Solid Edge part; units mm, degrees
sketch "Sketch1" plane through (-100.203, 10.668, -35.941) normal (0, 0, 1) x (-1, 0, 0)
  line L0 (4.1402, -5.9309) -> (4.1402, 5.9309)
  line L1 (4.1402, 5.9309) -> (-9.6647, 5.9309)
  line L2 (-9.6647, 5.9309) -> (-9.6647, -5.9309)
  line L3 (-9.6647, -5.9309) -> (4.1402, -5.9309)
extrude "Protrusion1" add sketch "Sketch1" along normal blind 5.334
sketch "Sketch2" plane through (-97.4407, 16.5989, -33.274) normal (0, 1, 0) x (-1, 0, 0)
  line L0 (4.9721, 2.9711) -> (3.1941, 2.9711)
  line L1 (3.1941, 2.9711) -> (3.1941, -1.3462)
  line L2 (3.1941, -1.3462) -> (4.9721, -1.3462)
  line L3 (4.9721, -1.3462) -> (4.9721, 2.9711)
extrude "Cutout1" cut sketch "Sketch2" against normal through all
sketch "Sketch3" plane through (-97.4407, 16.5989, -33.274) normal (0, 1, 0) x (-1, 0, 0)
  line L0 (0.6541, -1.6616) -> (-6.9024, -1.6616)
  line L1 (-6.9024, -1.6616) -> (-6.9024, -2.667)
  line L2 (-6.9024, -2.667) -> (0.6541, -2.667)
  line L3 (0.6541, -2.667) -> (0.6541, -1.6616)
extrude "Cutout2" cut sketch "Sketch3" against normal through all
fillet "Round_1" radius 0.8636 4 edges at (-104.3432, 10.668, -30.607) (-102.4128, 10.668, -30.607) (-100.6348, 10.668, -30.607) (-90.5383, 10.668, -30.607)
properties material "Gold"
Verification items for the finished model (mm, model axes). A direction names the side the tool comes from. Round coordinates to 2 decimals unless told otherwise and drop trailing zeros. Loops run counter-clockwise (first coordinate to the right, second up) from the corner with the lowest first, then second, coordinate; pieces in that order, holes last. Notation, with made-up numbers: (-14, 39.5) - (23, 39.5) arc R12 cw to (23, 56.5) - close; hole circle Ø8 at (-16.5, 25.25). An arc over 180 degrees is marked (long way). Answer in a Markdown table with one row per item. Add a question column.
Q1. Gauge pin test, flat ends, axial feed: pin 1 (2.5 mm diameter, centred on x = -94, y = 12, fed in from -Z); pin 2 (0.5 mm diameter, centred on x = -101, y = 10.5, fed in from +Z); pin 3 (0.8 mm diameter, centred on y = 12.5, z = -35.5, fed in from +X). Record the tip position at first contact, or that the pin passes through.
Q2. Section check B-B on y = 13. Enter the section's corners in (x, z), plus the area to 3 significant figures.
Q3. Release check for a two-part mould opening along X. For faces 1 (the face through (-97, 16.599, -33)), 2 (the face through (-102, 11, -34.62)), 3 (the face through (-104.08, 10.58, -30.85)) record: pulls with the +X half, pulls with the -X half, needs draft (parallel to the pull), parting line crosses it, or undercut.
Q4. Section check A-A on z = -34.45. Enter the section's corners in (x, y).
Q5. Tool access check on faces 4 (the face through (-102.413, 11, -33)), 5 (the face through (-98.095, 10.8, -35.4)), 6 (the face through (-90.538, 11, -33)). Record the directions out of +Z, -Z, +X, -X, +Y, -Y that give a thin tool (end or side, any length) a straight path to the whole face; none if there is none.
Q6. Material ranges on line 1 (X direction, y = 13, z = -31.9); line 2 (Z direction, x = -96, y = 8.75); line 3 (X direction, y = 14.75, z = -35.4), recorded low to high.
Q7. Section check D-D on z = -31.1. Enter the section's corners in (x, y), plus the area to 3 significant figures.
Q8. Section check C-C on x = -97.75. Enter the section's corners in (y, z), plus the area to 3 significant figures.
Found:
| question | item | result |
|---|---|---|
| 1 | pin 1 | stops at z = -34.94 |
| 1 | pin 2 | stops at z = -34.62 |
| 1 | pin 3 | stops at x = -98.09 |
| 2 | outline | (-104.34, -35.94) - (-98.09, -35.94) - (-98.09, -34.94) - (-90.54, -34.94) - (-90.54, -31.47) arc R0.86 ccw to (-91.4, -30.61) - (-99.77, -30.61) arc R0.86 ccw to (-100.63, -31.47) - (-100.63, -34.62) - (-102.41, -34.62) - (-102.41, -31.47) arc R0.86 ccw to (-103.28, -30.61) - (-103.48, -30.61) arc R0.86 ccw to (-104.34, -31.47) - close |
| 2 | area | 58.3 mm² |
| 3 | face 1 | needs draft |
| 3 | face 2 | undercut |
| 3 | face 3 | pulls with the -X half |
| 4 | outline | (-104.34, 4.74) - (-102.41, 4.74) - (-102.41, 16.6) - (-104.34, 16.6) - close; (-100.63, 4.74) - (-90.54, 4.74) - (-90.54, 16.6) - (-100.63, 16.6) - close |
| 5 | face 4 | +Z, +Y, -Y |
| 5 | face 5 | -Z, +X, +Y, -Y |
| 5 | face 6 | +Z, -Z, +X, +Y, -Y |
| 6 | line 1 | x = -104.34 to -102.41, -100.63 to -90.54 |
| 6 | line 2 | z = -34.94 to -30.61 |
| 6 | line 3 | x = -104.34 to -98.09 |
| 7 | outline | (-104.26, 4.74) - (-102.5, 4.74) - (-102.5, 16.6) - (-104.26, 16.6) - close; (-100.55, 4.74) - (-90.62, 4.74) - (-90.62, 16.6) - (-100.55, 16.6) - close |
| 7 | area | 139 mm² |
| 8 | outline | (4.74, -34.94) - (16.6, -34.94) - (16.6, -30.61) - (4.74, -30.61) - close |
| 8 | area | 51.3 mm² |
